Verification items for the finished model (mm, model axes). Round coordinates to 2 decimals unless told otherwise and drop trailing zeros. Loops run counter-clockwise (first coordinate to the right, second up) from the corner with the lowest first, then second, coordinate; pieces in that order, holes last. Notation, with made-up numbers: (55.5, 82.25) -> (64.5, 82.25) arc R10 cw to (64.5, 87.25) -> close; hole circle Ø10 at (27.5, -39). An arc over 180 degrees is marked (long way). Write item = value, one per line.
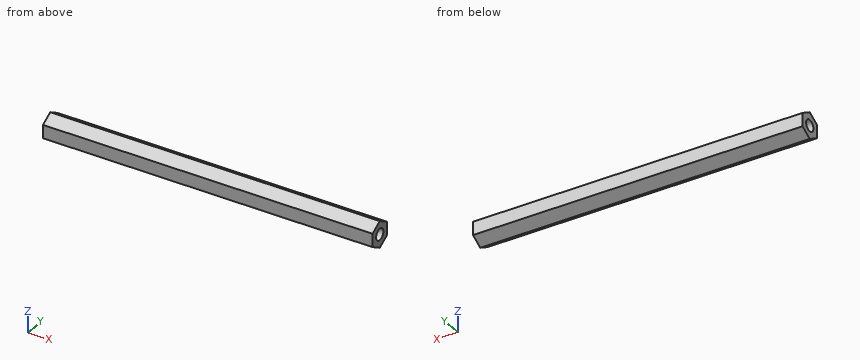
```python
from build123d import *

# Parameters (mm, degrees)
BOSS_EXTRUDE1_DEPTH       = 71.755
M3X0_5_TAPPED_HOLE1_D     = 2.5
M3X0_5_TAPPED_HOLE1_DEPTH = 7.493
M3X0_5_TAPPED_HOLE1_TIP   = 0.751075774
M3X0_5_TAPPED_HOLE2_D     = 2.5
M3X0_5_TAPPED_HOLE2_DEPTH = 7.493
M3X0_5_TAPPED_HOLE2_TIP   = 0.751075774


with BuildPart() as part:
    # Sketch1 → Boss-Extrude1 (new body)
    with BuildSketch(Plane(origin=(0, 0, 0), x_dir=(0, 0, -1), z_dir=(1, 0, 0))):
        Polygon((1.443375673, 2.5), (-1.443375673, 2.5), (-2.886751346, 0), (-1.443375673, -2.5), (1.443375673, -2.5), (2.886751346, 0), align=None)
    extrude(amount=BOSS_EXTRUDE1_DEPTH)

    # M3x0.5 Tapped Hole1
    with Locations(Plane.ZY):
        with Locations((0, 0)):
            Hole(M3X0_5_TAPPED_HOLE1_D / 2, depth=M3X0_5_TAPPED_HOLE1_DEPTH)
            with Locations((0, 0, -(M3X0_5_TAPPED_HOLE1_DEPTH + M3X0_5_TAPPED_HOLE1_TIP / 2))):  # 118° drill point
                Cone(0, M3X0_5_TAPPED_HOLE1_D / 2, M3X0_5_TAPPED_HOLE1_TIP, mode=Mode.SUBTRACT)

    # M3x0.5 Tapped Hole2
    with Locations(Plane(origin=(71.755, 0, 0), x_dir=(0, 0, -1), z_dir=(1, 0, 0))):
        with Locations((0, 0)):
            Hole(M3X0_5_TAPPED_HOLE2_D / 2, depth=M3X0_5_TAPPED_HOLE2_DEPTH)
            with Locations((0, 0, -(M3X0_5_TAPPED_HOLE2_DEPTH + M3X0_5_TAPPED_HOLE2_TIP / 2))):  # 118° drill point
                Cone(0, M3X0_5_TAPPED_HOLE2_D / 2, M3X0_5_TAPPED_HOLE2_TIP, mode=Mode.SUBTRACT)


solid = part.part
```
(1) Material ranges on probe 1 along Z at (x, y) = (3.5, 0); probe 2 along Y at (x, z) = (68.75, 0); probe 3 along Y at (x, z) = (5.5, -0.55), recorded low to high. Write a range as from..to.
Filled sheet:
probe_1 = -2.89..-1.25, 1.25..2.89
probe_2 = -2.5..-1.25, 1.25..2.5
probe_3 = -2.5..-1.12, 1.12..2.5
(2) Go/stop test with flat-tipped pins: pin 1 Ø1.5 at (y, z) = (-1, -0.5) entering from +X (3 decimals); pin 2 Ø2 at (y, z) = (0, 0) entering from +X. Record where each tip stops, or that it passes through.
Filled sheet:
pin_1 = 71.755
pin_2 = 64.11
(3) Sectioned sample at A-A, the plane x = 14. Record the cut outline in (y, z), and give its area (3 significant figures).
Filled sheet:
outline = (-2.5, -1.44) -> (0, -2.89) -> (2.5, -1.44) -> (2.5, 1.44) -> (0, 2.89) -> (-2.5, 1.44) -> close
area = 21.7 mm2
